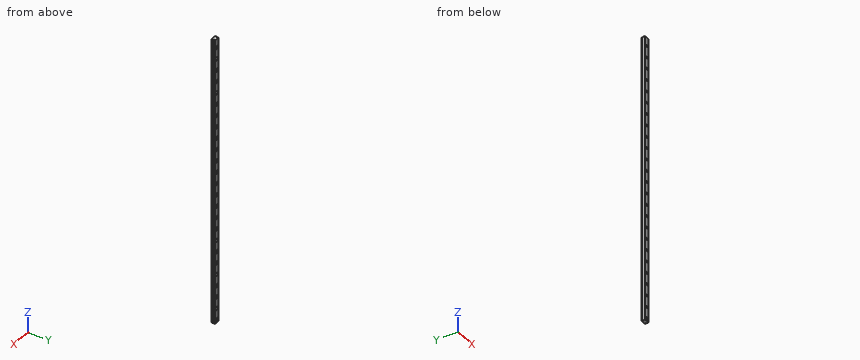
from build123d import *

# Parameters (mm, degrees)
EXTRUDE1_DEPTH  = 500
SKETCH2_R       = 3
EXTRUDE2_DEPTH  = 3.5
SKETCH_R        = 1.75
EXTRUDE3_DEPTH  = 7
LPATTERN1_COUNT = 30
LPATTERN1_PITCH = 20


with BuildPart() as part:
    # Sketch1 → Extrude1 (new body)
    with BuildSketch(Plane.XY):
        with BuildLine():
            Line((-4.5, -3), (4.5, -3))
            Line((4.5, -3), (4.5, 0))
            ThreePointArc((4.5, 0), (3.93077967, 0.177814974), (3.563991137, 0.648023568))
            Line((3.563991137, 0.648023568), (3.235073025, 0.648023568))
            Line((3.235073025, 0.648023568), (3.235073025, 1.351976432))
            Line((3.235073025, 1.351976432), (3.563991137, 1.351976432))
            ThreePointArc((3.563991137, 1.351976432), (3.93077967, 1.822185026), (4.5, 2))
            Line((4.5, 2), (4.5, 3))
            Line((4.5, 3), (-4.5, 3))
            Line((-4.5, 3), (-4.5, 2))
            ThreePointArc((-4.5, 2), (-3.93077967, 1.822185026), (-3.563991137, 1.351976432))
            Line((-3.563991137, 1.351976432), (-3.235073025, 1.351976432))
            Line((-3.235073025, 1.351976432), (-3.235073025, 0.648023568))
            Line((-3.235073025, 0.648023568), (-3.563991137, 0.648023568))
            ThreePointArc((-3.563991137, 0.648023568), (-3.93077967, 0.177814974), (-4.5, 0))
            Line((-4.5, 0), (-4.5, -3))
        make_face()
    extrude(amount=EXTRUDE1_DEPTH)

    # Sketch2 → Extrude2 (cut)
    with BuildSketch(Plane(origin=(0, 3, 0), x_dir=(1, 0, 0), z_dir=(0, 1, 0))):
        with Locations((0, -5)):
            Circle(SKETCH2_R)
    extrude2 = extrude(amount=-EXTRUDE2_DEPTH, mode=Mode.SUBTRACT)

    # Sketch → Extrude3 (cut, through all)
    with BuildSketch(Plane(origin=(0, 3, 0), x_dir=(1, 0, 0), z_dir=(0, 1, 0))):
        with Locations((0, -5)):
            Circle(SKETCH_R)
    extrude3 = extrude(amount=-EXTRUDE3_DEPTH, mode=Mode.SUBTRACT)

    # LPattern1: Extrude2, Extrude3 ×30
    with Locations(*[(0, 0, i * LPATTERN1_PITCH) for i in range(1, LPATTERN1_COUNT)]):
        add(extrude2, mode=Mode.SUBTRACT)
        add(extrude3, mode=Mode.SUBTRACT)


solid = part.part
For this review, take the finished solid that the model builds, in its own axes (mm). Round coordinates to 2 decimals unless told otherwise and drop trailing zeros. Answer as CSV lines item,"result".
(1) Wall thickness on line 1 (X direction, y = 0.9, z = 345); line 2 (X direction, y = 2.25, z = 265); line 3 (Y direction, x = 1, z = 103): over which ranges is each line inside the solid? List them lowest first.
Checked values:
line 1,"x = -3.24 to -3, 3 to 3.24"
line 2,"x = -4.5 to -3, 3 to 4.5"
line 3,"y = -3 to -0.5"
(2) Consider section A-A on x = 0. Give the number of separate pieces and of enclosed holes in the cut face, then the cut area to 3 significant figures.
Checked values:
separate pieces,"26"
enclosed holes,"0"
area,"2,260 mm2"
(3) Insertion check: P1, Ø3, axis at x = 0, z = 305, coming from the +Y side; P2, Ø3, axis at x = -0.5, z = 246, coming from the +Y side. Each pin has a flat end and moves straight along its axis. Give the tip position at first contact, or say it passes through.
Checked values:
P1,"passes through"
P2,"stops at y = -0.5"
